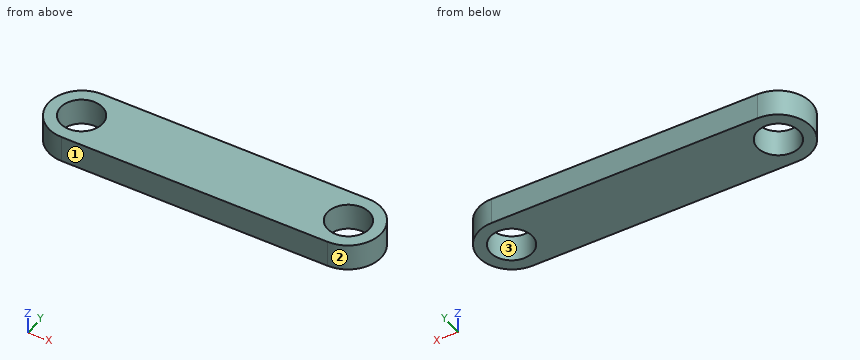
from build123d import *

# Parameters (mm, degrees)
SKETCH1_R           = 2.395
BOSS_EXTRUDE1_DEPTH = 3
SKETCH2_R           = 2.365
BOSS_EXTRUDE2_DEPTH = 3


with BuildPart() as part:
    # Sketch1 → Boss-Extrude1 (new body)
    with BuildSketch(Plane.XY):
        with BuildLine():
            Line((0, 3), (30, 3))
            ThreePointArc((30, 3), (33, 0), (30, -3))
            Line((30, -3), (0, -3))
            ThreePointArc((0, -3), (-3, 0), (0, 3))
        make_face()
        Circle(SKETCH1_R, mode=Mode.SUBTRACT)
        with Locations((30, 0)):
            Circle(SKETCH1_R, mode=Mode.SUBTRACT)
    extrude(amount=BOSS_EXTRUDE1_DEPTH)

    # Sketch2 → Boss-Extrude2 (add)
    with BuildSketch(Plane.XY.offset(3)):
        with BuildLine():
            Line((0.05, 3.75), (29.95, 3.75))
            ThreePointArc((29.95, 3.75), (33.7, 0), (29.95, -3.75))
            Line((29.95, -3.75), (0.05, -3.75))
            ThreePointArc((0.05, -3.75), (-3.7, 0), (0.05, 3.75))
        make_face()
        Circle(SKETCH2_R, mode=Mode.SUBTRACT)
        with Locations((30, 0)):
            Circle(SKETCH2_R, mode=Mode.SUBTRACT)
    extrude(amount=-BOSS_EXTRUDE2_DEPTH)


solid = part.part
For this review, take the finished solid that the model builds, in its own axes (mm). Face numbers are marked on the shaded views. Round coordinates to 2 decimals unless told otherwise and drop trailing zeros. Loops run counter-clockwise (first coordinate to the right, second up) from the corner with the lowest first, then second, coordinate; pieces in that order, holes last. Notation, with made-up numbers: (-2.75, 85) - (6.25, 85) arc R6 ccw to (6.25, 93) - close; hole circle Ø3 at (50.25, 29). An arc over 180 degrees is marked (long way). Use one line per item in the form item = value.
Item 1: Consider section D-D on y = -1.5. Write out the cut boundary in (x, z).
Answers:
outline = (-3.39, 0) - (-1.83, 0) - (-1.83, 3) - (-3.39, 3) - close; (1.83, 0) - (28.17, 0) - (28.17, 3) - (1.83, 3) - close; (31.83, 0) - (33.39, 0) - (33.39, 3) - (31.83, 3) - close
Item 2: Consider section C-C on x = 2. Write out the cut boundary in (y, z), then the cut area to 3 significant figures.
Answers:
outline = (-3.75, 0) - (-1.26, 0) - (-1.26, 3) - (-3.75, 3) - close; (1.26, 0) - (3.75, 0) - (3.75, 3) - (1.26, 3) - close
area = 14.9 mm^2
Item 3: Mouldability with a two-part tool opening along Y and no side actions: class the marked faces 1, 2 and 3 as +Y half, -Y half, draft (parallel to the pull), parting line (faces both ways), or undercut.
Answers:
face_1 = -Y half
face_2 = parting line
face_3 = undercut
Item 4: Clearance check with flat-ended pins moving along their axes: P1, Ø3, axis at x = 0, y = 0, coming from the -Z side; P2, Ø1.5, axis at y = 2, z = 2.5, coming from the -X side. State where each tip first meets the part, or that it passes through.
Answers:
P1 = through
P2 = -3.49
Item 5: For line 1 (X direction, y = -0.5, z = 2.2); line 2 (Y direction, x = 30, z = 2.2) (3 decimals); line 3 (Y direction, x = 30.5, z = 0.9), list the stretches that pass through material, from the lowest coordinate up.
Answers:
line_1 = -3.67 to -2.31, 2.31 to 27.69, 32.31 to 33.67
line_2 = -3.75 to -2.365, 2.365 to 3.75
line_3 = -3.71 to -2.31, 2.31 to 3.71
Item 6: Consider section B-B on z = 0.5. Write out the cut boundary in (x, y) (3 decimals).
Answers:
outline = (0.05, -3.75) - (29.95, -3.75) arc R3.75 ccw to (29.95, 3.75) - (0.05, 3.75) arc R3.75 ccw to start; hole circle Ø4.73 at (0, 0); hole circle Ø4.73 at (30, 0)
Item 7: Consider section A-A on y = 0. Write out the cut boundary in (x, z) (3 decimals), then the cut area to 3 significant figures.
Answers:
outline = (-3.7, 0) - (-2.365, 0) - (-2.365, 3) - (-3.7, 3) - close; (2.365, 0) - (27.635, 0) - (27.635, 3) - (2.365, 3) - close; (32.365, 0) - (33.7, 0) - (33.7, 3) - (32.365, 3) - close
area = 83.8 mm^2
